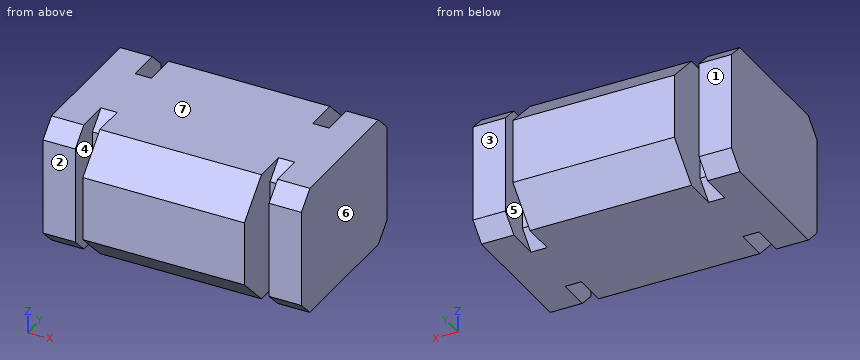
```python
from build123d import *

# Parameters (mm, degrees)
F1_DEPTH = 8
F2_SIZE  = 1
F3_SIZE  = 2


with BuildPart() as f1:
    # F0 (on Top) → F1 (new body)
    with BuildSketch(Plane.XY):
        Polygon((5, 6), (0, 6), (-5, 6), (-5, 3), (-6, 3), (-6, 5), (-8, 5), (-8, -5), (-6, -5), (-6, -3), (-5, -3), (-5, -6), (0, -6), (5, -6), (5, -3), (6, -3), (6, -5), (8, -5), (8, 5), (6, 5), (6, 3), (5, 3), align=None)
    extrude(amount=F1_DEPTH)

    # F2
    f2_edges = [f1.edges().sort_by_distance(p)[0] for p in [
        (-7, -5, 0),
        (-7, 5, 0),
        (7, -5, 0),
        (7, 5, 0),
        (-7, -5, 8),
        (-7, 5, 8),
        (7, -5, 8),
        (7, 5, 8),
        (5.5, -3, 8),
        (5.5, 3, 8),
        (-5.5, -3, 8),
        (-5.5, 3, 8),
        (-5.5, -3, 0),
        (-5.5, 3, 0),
        (5.5, 3, 0),
        (5.5, -3, 0),
    ]]
    chamfer(f2_edges, length=F2_SIZE)

    # F3
    f3_edges = [f1.edges().sort_by_distance(p)[0] for p in [
        (0, -6, 8),
        (0, -6, 0),
        (0, 6, 8),
        (0, 6, 0),
    ]]
    chamfer(f3_edges, length=F3_SIZE)


solid = f1.part
```
CAD build for the part. Positions are in the model's coordinates, mm. Face numbers are marked on the shaded views. A direction names the side the tool comes from. Coordinates: 2 decimals unless noted, no trailing zeros. Order: outer loops, then holes, each group sorted by start corner. A loop starts at its lowest first (then second) coordinate and runs counter-clockwise, first axis right, second up.
(1) Mould opens along X. For the marked faces 4, 5, 6 and 7 say: released by +X, released by -X, zero draft, split by the parting line, or undercut.
Solution:
face 4: undercut
face 5: undercut
face 6: released by +X
face 7: zero draft
(2) Saw through at D-D, the plane y = -4.5. Write the cut outline in (x, z).
Solution:
outline: (-8, 0.5) - (-6, 0.5) - (-6, 7.5) - (-8, 7.5) - close; (-5, 0.5) - (5, 0.5) - (5, 7.5) - (-5, 7.5) - close; (6, 0.5) - (8, 0.5) - (8, 7.5) - (6, 7.5) - close
(3) Saw through at B-B, the plane x = -4.25. Write the cut outline in (y, z).
Solution:
outline: (-6, 2) - (-4, 0) - (4, 0) - (6, 2) - (6, 6) - (4, 8) - (-4, 8) - (-6, 6) - close
(4) Drill centre lines: L1, parallel to X at y = -3.75, z = 4.5; L2, parallel to Y at x = 0.75, z = 1; L3, parallel to Y at x = -5.75, z = 4.5. Where is each one in solid material? Low to high.
Solution:
L1: x = -8 to -6, -5 to 5, 6 to 8
L2: y = -5 to 5
L3: y = -3 to 3
(5) Which spindle directions (+Z, -Z, +X, -X, +Y, -Y) get a long thin tool onto all of the face, cutting with end or side? Do the marked faces 1, 2 and 3. Say none if no direction does.
Solution:
face 1: +Z, -Z, -X, +Y
face 2: +Z, -Z, -X, -Y
face 3: +Z, -Z, +X, +Y
(6) Saw through at C-C, the plane z = 6.5. Write the cut outline in (x, y).
Solution:
outline: (-8, -5) - (-6, -5) - (-6, -3) - (-5, -3) - (-5, -5.5) - (5, -5.5) - (5, -3) - (6, -3) - (6, -5) - (8, -5) - (8, 5) - (6, 5) - (6, 3) - (5, 3) - (5, 5.5) - (-5, 5.5) - (-5, 3) - (-6, 3) - (-6, 5) - (-8, 5) - close
(7) Pin check, flat tips, straight feed: pin 1 Ø1 at (x, z) = (6.5, 4.5) entering from +Y; pin 2 Ø0.8 at (x, z) = (5.5, 5.5) entering from +Y; pin 3 Ø1.6 at (x, z) = (7.5, 5) entering from -Y. Stop position of each tip, or through.
Solution:
pin 1: stops at y = 5
pin 2: stops at y = 3
pin 3: stops at y = -5
(8) Saw through at A-A, the plane y = 3.5. Write the cut outline in (x, z).
Solution:
outline: (-8, 0) - (-6, 0) - (-6, 8) - (-8, 8) - close; (-5, 0) - (5, 0) - (5, 8) - (-5, 8) - close; (6, 0) - (8, 0) - (8, 8) - (6, 8) - close
